For this review, take the finished solid that the model builds, in its own axes (mm). Coordinates: 2 decimals unless noted, no trailing zeros. Loops run counter-clockwise (first coordinate to the right, second up) from the corner with the lowest first, then second, coordinate; pieces in that order, holes last. Notation, with made-up numbers: (59, 48) - (91, 48) arc R20 cw to (91, 57) - close; hole circle Ø2 at (31.5, 30). An arc over 180 degrees is marked (long way). One line per item, written item: value. Start each with the question number.
1. Take a section at D-D, the plane z = 1.05. State the section outline as (x, y) points.
2. To check wall thickness, follow line 1 (Z direction, x = -3.5, y = -1.6); line 2 (Y direction, x = -3.25, z = -0.1); line 3 (Y direction, x = -5, z = -1.05). State the ranges of each line that lie inside material, in increasing order. Write a range as from..to.
3. Take a section at A-A, the plane y = 0. State the section outline as (x, z) points.
4. Insertion check: pin 1 (2 mm diameter, centred on y = -1.5, z = -0.5, fed in from -X). The pin has a flat end and moves straight along its axis. Give the tip position at first contact, or say it passes through.
5. Take a section at C-C, the plane z = -1.6. State the section outline as (x, y) points.
6. Take a section at B-B, the plane x = -0.25. State the section outline as (y, z) points, and give its area (3 significant figures).
```python
from build123d import *

# Parameters (mm, degrees)
F1_DEPTH      = 1.29
F1_DEPTH_BACK = 2.67
F2_R          = 1.29


with BuildPart() as f1:
    # F0 (on Top) → F1 (new body, two sides)
    with BuildSketch(Plane.XY) as f1_sk:
        with BuildLine():
            Line((3.11, 2.88), (-3.11, 2.88))
            ThreePointArc((-3.11, 2.88), (-5.99, 0), (-3.11, -2.88))
            Line((-3.11, -2.88), (3.11, -2.88))
            ThreePointArc((3.11, -2.88), (5.99, 0), (3.11, 2.88))
        make_face()
    extrude(amount=F1_DEPTH)
    extrude(f1_sk.sketch, amount=-F1_DEPTH_BACK)

    # F2
    f2_edges = [f1.edges().sort_by_distance(p)[0] for p in [
        (5.99, 0, 1.29),
        (0, 2.88, 1.29),
        (0, -2.88, 1.29),
        (-5.99, 0, 1.29),
    ]]
    fillet(f2_edges, radius=F2_R)


solid = f1.part
```
Solutions:
1. outline: (-3.11, -2.34) - (3.11, -2.34) arc R2.34 ccw to (3.11, 2.34) - (-3.11, 2.34) arc R2.34 ccw to start
2. line 1: -2.67..1.29
2. line 2: -2.88..2.88
2. line 3: -2.17..2.17
3. outline: (-5.99, -2.67) - (5.99, -2.67) - (5.99, 0) arc R1.29 ccw to (4.7, 1.29) - (-4.7, 1.29) arc R1.29 ccw to (-5.99, 0) - close
4. pin 1: x = -5.95
5. outline: (-3.11, -2.88) - (3.11, -2.88) arc R2.88 ccw to (3.11, 2.88) - (-3.11, 2.88) arc R2.88 ccw to start
6. outline: (-2.88, -2.67) - (2.88, -2.67) - (2.88, 0) arc R1.29 ccw to (1.59, 1.29) - (-1.59, 1.29) arc R1.29 ccw to (-2.88, 0) - close
6. area: 22.1 mm2
